Part model, mm, in its own coordinate system. A direction names the side the tool comes from. Give positions to 0.01 mm unless a question says otherwise; leave off trailing zeros. Write each loop counter-clockwise with the first axis right and the second up, starting at its lowest first coordinate (ties: lowest second). Pieces come first, ordered by that corner, then holes.
from build123d import *

# Parameters (mm, degrees)
CUT_EXTRUDE1_DEPTH = 21
SKETCH5_W          = 19.327905808
SKETCH5_H          = 9.031167277
CUT_EXTRUDE4_DEPTH = 25
CUT_EXTRUDE5_DEPTH = 5
SKETCH9_R          = 2
CUT_EXTRUDE6_DEPTH = 10
SKETCH10_R         = 2.5
CUT_EXTRUDE7_DEPTH = 10


with BuildPart() as part:
    # Sketch1 → Revolve1 (revolve)
    with BuildSketch(Plane(origin=(0, 0, 0), x_dir=(1, 0, 0), z_dir=(0, 1, 0))):
        Polygon((0, 0), (0, 6.5), (116, 6.5), (120, 5), (131, 5), (131, 3.5), (268, 3.5), (268, 0), align=None)
    revolve(axis=Axis((0, 0, 0), (1, 0, 0)))

    # Sketch2 → Cut-Extrude1 (cut, symmetric)
    with BuildSketch(Plane(origin=(0, 0, 0), x_dir=(1, 0, 0), z_dir=(0, 1, 0))):
        with BuildLine():
            Line((0, 6.5), (0, 2.5))
            Line((0, 2.5), (16, 2.5))
            ThreePointArc((16, 2.5), (18.611709863, 5.082435206), (22, 6.5))
            Line((22, 6.5), (0, 6.5))
        make_face()
        with BuildLine():
            Line((16, -2.5), (0, -2.5))
            Line((0, -2.5), (0, -6.5))
            Line((0, -6.5), (22, -6.5))
            ThreePointArc((22, -6.5), (18.611709863, -5.082435206), (16, -2.5))
        make_face()
    extrude(amount=CUT_EXTRUDE1_DEPTH, both=True, mode=Mode.SUBTRACT)

    # Sketch5 → Cut-Extrude4 (cut)
    with BuildSketch(Plane(origin=(0, 0, -2.5), x_dir=(-1, 0, 0), z_dir=(0, 0, -1))):
        with Locations((-6.336047096, 10.515583639)):
            Rectangle(SKETCH5_W, SKETCH5_H)
    extrude(amount=-CUT_EXTRUDE4_DEPTH, mode=Mode.SUBTRACT)

    # Sketch8 → Cut-Extrude5 (cut, symmetric)
    with BuildSketch(Plane.XY):
        Polygon((250, 2), (275.037154833, 2), (275.037154833, 6.622106016), (250, 7.374727948), align=None)
        Polygon((275.037154833, -10.204370032), (275.037154833, -2), (250, -2), (250, -8.806643588), align=None)
    extrude(amount=CUT_EXTRUDE5_DEPTH, both=True, mode=Mode.SUBTRACT)

    # Sketch9 → Cut-Extrude6 (cut)
    with BuildSketch(Plane(origin=(0, 2, 0), x_dir=(1, 0, 0), z_dir=(0, 1, 0))):
        with Locations((258.568042263, 0)):
            Circle(SKETCH9_R)
    extrude(amount=-CUT_EXTRUDE6_DEPTH, mode=Mode.SUBTRACT)

    # Sketch10 → Cut-Extrude7 (cut)
    with BuildSketch(Plane.XY.offset(2.5)):
        with Locations((8, 0)):
            Circle(SKETCH10_R)
    extrude(amount=-CUT_EXTRUDE7_DEPTH, mode=Mode.SUBTRACT)


solid = part.part
1) Saw through at D-D (x = 107.5). Write the cut outline in (y, z), and give its area (3 significant figures).
Check result:
outline: circle Ø13 at (0, 0)
area: 133 mm2
2) Mould opens along Y. For faces 1 (the flat face through (131, -3.3, -2.2)), 2 (the cylindrical face through (10.385, 0.751, 0.035)), 3 (the cylindrical face through (71.701, -3.955, 5.158)) say: +Y half, -Y half, draft (parallel to the pull), parting line (faces both ways), or undercut.
Check result:
face 1: draft
face 2: undercut
face 3: parting line
3) Flat gauge pins, fed straight in: P1, Ø4, axis at x = 201.5, z = -1.5, coming from the -Y side; P2, Ø6.5, axis at x = 260, z = 1, coming from the +Y side; P3, Ø6, axis at x = 9, y = 2, coming from the +Z side; P4, Ø4.5, axis at x = 8, y = 0, coming from the +Z side. Where does each tip first touch, or does it go through?
Check result:
P1: stops at y = -3.5
P2: stops at y = 2
P3: stops at z = 2.5
P4: passes through
4) Drill centre lines: L1, parallel to X at y = -0.4, z = 0; L2, parallel to Y at x = 8, z = 0.65; L3, parallel to X at y = 1.5, z = -1.5. Where is each one in solid material? Low to high.
Check result:
L1: x = 0 to 5.53, 10.47 to 256.57, 260.57 to 268
L2: y = -6.47 to -2.5, 2.5 to 6
L3: x = 0 to 6, 10 to 257.25, 259.89 to 268
5) 3-axis set-ups, long thin cutter, end or side, ignore diameter. For faces 4 (the flat face through (261, -2, 0)), 5 (the flat face through (8, 3, 2.5)), 6 (the cylindrical face through (125.58, -4.88, 1.08)), 7 (the flat face through (8, -3, -2.5)): which of +Z, -Z, +X, -X, +Y, -Y reach the whole face in a straight line?
Check result:
face 4: +Z, -Z, +X, -Y
face 5: +Z, -X, +Y, -Y
face 6: +X
face 7: -Z, -X, +Y, -Y
6) Saw through at A-A (y = 0). Write the cut outline in (x, z), and give its area (3 significant figures).
Check result:
outline: (0, -2.5) - (5.5, -2.5) - (5.5, 2.5) - (0, 2.5) - close; (10.5, -2.5) - (16, -2.5) arc R9.64 ccw to (22, -6.5) - (116, -6.5) - (120, -5) - (131, -5) - (131, -3.5) - (268, -3.5) - (268, 3.5) - (131, 3.5) - (131, 5) - (120, 5) - (116, 6.5) - (22, 6.5) arc R9.64 ccw to (16, 2.5) - (10.5, 2.5) - close; hole circle Ø4 at (258.57, 0)
area: 2,440 mm2
7) Saw through at C-C (x = 8). Write the cut outline in (y, z), and give its area (3 significant figures).
Check result:
outline: (-6, -2.5) - (-2.5, -2.5) - (-2.5, 2.5) - (-6, 2.5) arc R6.5 ccw to start; (2.5, -2.5) - (6, -2.5) - (6, 2.5) - (2.5, 2.5) - close
area: 36.7 mm2
8) Saw through at B-B (z = 0). Write the cut outline in (x, y), and give its area (3 significant figures).
Check result:
outline: (0, -6.5) - (116, -6.5) - (120, -5) - (131, -5) - (131, -3.5) - (250, -3.5) - (250, -2) - (256.57, -2) - (256.57, 2) - (250, 2) - (250, 3.5) - (131, 3.5) - (131, 5) - (120, 5) - (116, 6.5) - (16, 6.5) - (16, 6) - (0, 6) - close; (260.57, -2) - (268, -2) - (268, 2) - (260.57, 2) - close; hole circle Ø5 at (8, 0)
area: 2,530 mm2
